Part model, mm, in its own coordinate system. Round coordinates to 2 decimals unless told otherwise and drop trailing zeros. Write each loop counter-clockwise with the first axis right and the second up, starting at its lowest first coordinate (ties: lowest second). Pieces come first, ordered by that corner, then holes. Notation, with made-up numbers: (-8.5, 20.25) -> (27.5, 20.25) arc R23 ccw to (27.5, 54.25) -> close; hole circle Ø1 at (89, 51.25). An arc over 180 degrees is marked (long way). Return JSON: item names as keys, results as strings. Group by question number.
```python
from build123d import *

# Parameters (mm, degrees)
F0_W     = 14
F0_H     = 14
F1_DEPTH = 44
F2_R     = 5
F3_R     = 5


with BuildPart() as f1:
    # F0 (on Top) → F1 (new body)
    with BuildSketch(Plane.XY):
        Rectangle(F0_W, F0_H)
    extrude(amount=F1_DEPTH)

    # F2
    f2_edges = [f1.edges().sort_by_distance(p)[0] for p in [
        (0, -7, 0),
        (0, 7, 0),
        (0, -7, 44),
        (0, 7, 44),
    ]]
    fillet(f2_edges, radius=F2_R)

    # F3
    f3_edges = [f1.edges().sort_by_distance(p)[0] for p in [
        (7, 7, 22),
        (0, 7, 5),
        (0, 7, 39),
        (-7, 7, 22),
    ]]
    fillet(f3_edges, radius=F3_R)


solid = f1.part
```
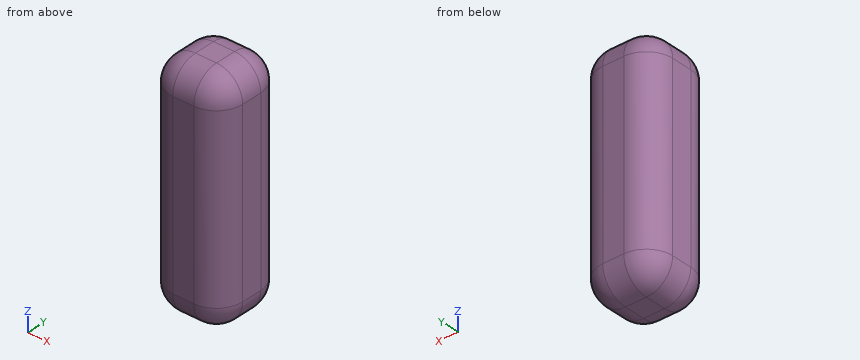
Item 1: Cut at B-B (y = -6). Write the cut outline in (x, z).
Item 2: Flat gauge pins, fed straight in: P1, Ø8, axis at x = -3, z = 28.5, coming from the -Y side; P2, Ø3, axis at x = 5, y = -0.5, coming from the +Z side. Where does each tip first touch, or does it go through?
Item 3: Wall check: L1, parallel to X at y = -2.25, z = 22; L2, parallel to Y at x = 4.75, z = 15.5; L3, parallel to X at y = 6, z = 39. Give the ranges that are in metal, low to high.
Item 4: Cut at A-A (z = 14). Write the cut outline in (x, y), then the cut area to 3 significant figures.
Checks:
{
 "1": {"outline": "(-5, 5) arc R3 ccw to (-2, 2) -> (2, 2) arc R3 ccw to (5, 5) -> (5, 39) arc R3 ccw to (2, 42) -> (-2, 42) arc R3 ccw to (-5, 39) -> close"},
 "2": {"P1": "stops at y = -7", "P2": "stops at z = 43.77"},
 "3": {"L1": "x = -6.99 to 6.99", "L2": "y = -6.18 to 6.18", "L3": "x = -5 to 5"},
 "4": {"outline": "(-7, -2) arc R5 ccw to (-2, -7) -> (2, -7) arc R5 ccw to (7, -2) -> (7, 2) arc R5 ccw to (2, 7) -> (-2, 7) arc R5 ccw to (-7, 2) -> close", "area": "175 mm2"}
}
